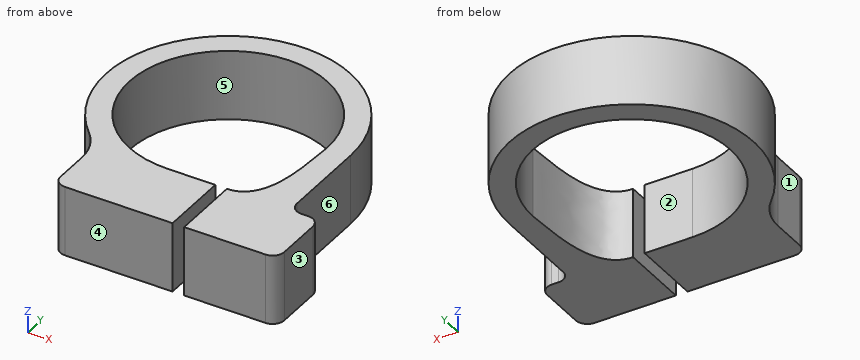
```python
from build123d import *

# Parameters (mm, degrees)
F1_DEPTH = 9.525


with BuildPart() as f1:
    # F0 (on Top) → F1 (new body)
    with BuildSketch(Plane.XY):
        with BuildLine():
            ThreePointArc((0, -13.49375), (-9.541522, 9.541522), (13.49375, 0))
            add(Edge.make_bspline(
                [(8.091652, -13.49375), (13.864147, -13.49375), (13.182361, -2.882126), (13.49375, 0)],
                knots=[0, 0, 0, 0, 14.534922, 14.534922, 14.534922, 14.534922], degree=3))
            Line((8.091652, -13.49375), (8.091652, -23.01875))
            Line((8.091652, -23.01875), (19.204152, -23.01875))
            ThreePointArc((19.204152, -23.01875), (20.326684, -22.553782), (20.791652, -21.43125))
            Line((20.791652, -21.43125), (20.791652, -15.08125))
            ThreePointArc((20.791652, -15.08125), (20.326684, -13.958718), (19.204152, -13.49375))
            Line((19.204152, -13.49375), (18.25625, -13.49375))
            ThreePointArc((18.25625, -13.49375), (17.133718, -13.028782), (16.66875, -11.90625))
            Line((16.66875, -11.90625), (16.66875, 0))
            ThreePointArc((16.66875, 0), (-6.378854, 15.399917), (-11.786586, -11.786586))
            ThreePointArc((-11.786586, -11.786586), (-10.289896, -14.026542), (-9.764328, -16.66875))
            Line((-9.764328, -16.66875), (-9.764328, -21.43125))
            ThreePointArc((-9.764328, -21.43125), (-9.29936, -22.553782), (-8.176828, -23.01875))
            Line((-8.176828, -23.01875), (6.504152, -23.01875))
            Line((6.504152, -23.01875), (6.504152, -13.49375))
            Line((6.504152, -13.49375), (0, -13.49375))
        make_face()
    extrude(amount=F1_DEPTH)


solid = f1.part
```
Could you check a few things on this model? Use its own coordinates, in mm. Face numbers are marked on the shaded views. A direction names the side the tool comes from. Coordinates: 2 decimals unless noted, no trailing zeros. Order: outer loops, then holes, each group sorted by start corner. A loop starts at its lowest first (then second) coordinate and runs counter-clockwise, first axis right, second up. Notation, with made-up numbers: M 10.25,69 L 26.25,69 A25 cw 26.25,83 Z; hole C -2,4 d2. An arc over 180 degrees is marked long. Use one line per item in the form item = value. Start each with the question number.
1. We'd pull the mould along X, two halves only. Please class the marked faces 4, 5 and 6: +X half, -X half, draft (parallel to the pull), parting line (faces both ways), or undercut.
2. Please list where these lines run through material, in increasing order: line 1 (Y direction, x = 0, z = 8.25); line 2 (X direction, y = -17.5, z = 1); line 3 (Y direction, x = 5, z = 8.5).
3. Suppose I cut it at B-B on y = 3. Write out the boundary of the cut face in (x, z) (3 decimals).
4. On a 3-axis mill with a long thin cutter (end or side, diameter ignored), from which of +Z, -Z, +X, -X, +Y, -Y can I reach the whole of each face in a straight line? I mean the marked faces 1, 2 and 3. Say none if no direction works.
5. Suppose I cut it at A-A on x = -11. Write out the boundary of the cut face in (y, z) (3 decimals), then the cut area to 3 significant figures.
6. For pin 1 (4 mm diameter, centred on x = 5.5, z = 4.5, fed in from +Y); pin 2 (1.5 mm diameter, centred on y = -4.5, z = 4, fed in from -X); pin 3 (16 mm diameter, centred on x = 0, y = 0, fed in from -Z); pin 4 (1.4 mm diameter, centred on y = -19.5, z = 6.5, fed in from -X), each with a flat end and sliding along its axis, tell me the tip position at first contact or that it passes through.
Geometry says:
q1.face_4 = draft
q1.face_5 = undercut
q1.face_6 = +X half
q2.line_1 = -23.02 to -13.49, 13.49 to 16.67
q2.line_2 = -9.76 to 6.5, 8.09 to 20.79
q2.line_3 = -23.02 to -13.49, 12.53 to 15.9
q3.outline = M -16.397,0 L -13.156,0 L -13.156,9.525 L -16.397,9.525 Z; M 13.156,0 L 16.397,0 L 16.397,9.525 L 13.156,9.525 Z
q4.face_1 = +Z, -Z, -X, -Y
q4.face_2 = +Z, -Z
q4.face_3 = +Z, -Z, +X, +Y, -Y
q5.outline = M -12.727,0 L -7.815,0 L -7.815,9.525 L -12.727,9.525 Z; M 7.815,0 L 12.524,0 L 12.524,9.525 L 7.815,9.525 Z
q5.area = 91.6 mm^2
q6.pin_1 = 16.3
q6.pin_2 = -16.24
q6.pin_3 = through
q6.pin_4 = -9.76
